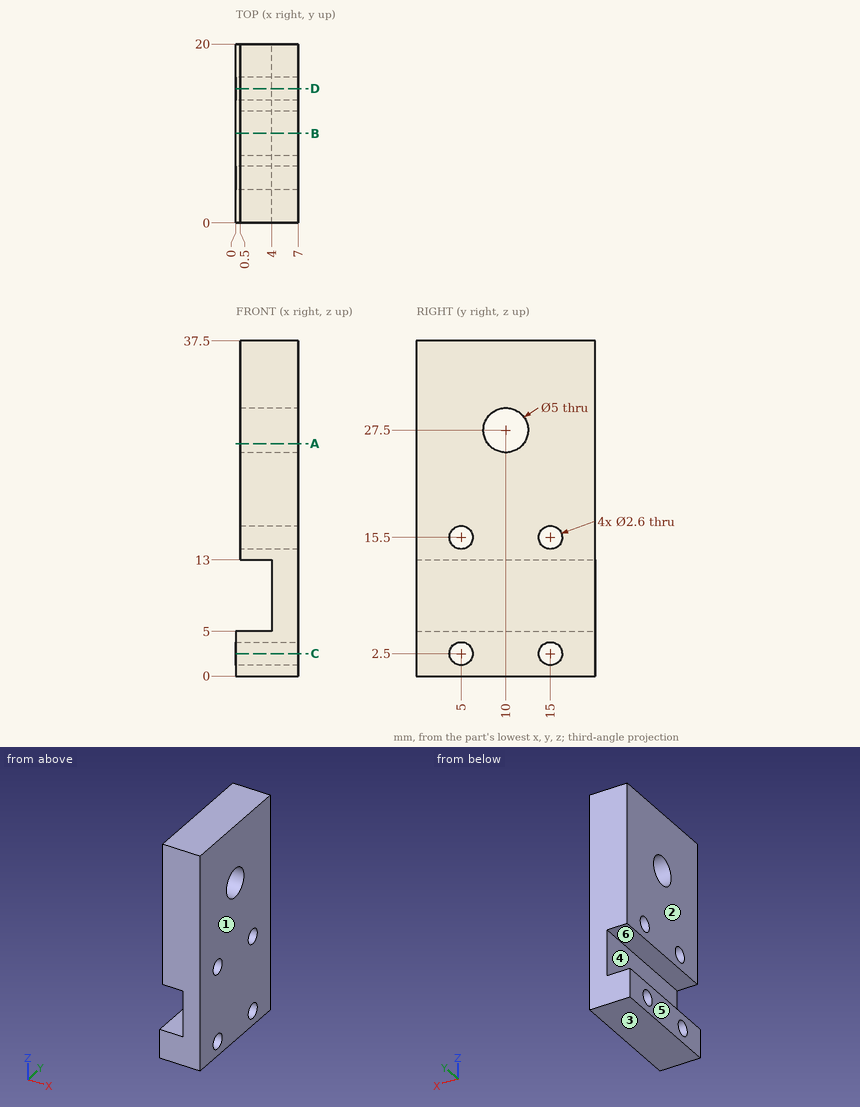
Could you check a few things on this drawing? It's one solid part, dimensions in mm from its lowest x, y, z. A direction names the side the tool comes from. Give positions to 0.01 mm unless a question says otherwise; leave off trailing zeros. Write each loop counter-clockwise with the first axis right and the second up, starting at its lowest first coordinate (ties: lowest second). Pieces come first, ordered by that corner, then holes. Notation, with made-up numbers: M 46,8.25 L 81,8.25 A29 cw 81,41.25 Z; hole C 76,11.5 d1. An arc over 180 degrees is marked long. Put each result on its own line as item: value. Start each with the question number.
Item 1: Thinking about a two-plate mould opening in Z: for the marked faces 3, 4, 5 and 6, which applies, +Z half, -Z half, draft (parallel to the pull), parting line (faces both ways), or undercut?
Item 2: If we section it at B-B, the plane y = 10: Write out the boundary of the cut face in (x, z), then the cut area to 3 significant figures.
Item 3: If we section it at A-A, the plane z = 26: Write out the boundary of the cut face in (x, y), then the cut area to 3 significant figures.
Item 4: On a 3-axis mill with a long thin cutter (end or side, diameter ignored), from which of +Z, -Z, +X, -X, +Y, -Y can I reach the whole of each face in a straight line? I mean the marked faces 1 and 2. Say none if no direction works.
Item 5: If we section it at D-D, the plane y = 15: Write out the boundary of the cut face in (x, z).
Item 6: Will these pins go through, and if not, where does the flat tip stop? pin 1 (8 mm diameter, centred on y = 9, z = 25, fed in from -X); pin 2 (4 mm diameter, centred on y = 12, z = 8, fed in from -X).
Item 7: If we section it at C-C, the plane z = 2.5: Write out the boundary of the cut face in (x, y), then the cut area to 3 significant figures.
Item 8: I need wall thicknesses on L1, parallel to Y at x = 2.5, z = 15.5; L2, parallel to Z at x = 2.25, y = 16.5; L3, parallel to Z at x = 5.25, y = 15.25. Which ranges of each line are inside material? Lowest first, please. Write a range as from..to.
Values:
1. face 3: -Z half
1. face 4: undercut
1. face 5: draft
1. face 6: undercut
2. outline: M 0,0 L 7,0 L 7,25 L 0.5,25 L 0.5,13 L 4,13 L 4,5 L 0,5 Z; M 0.5,30 L 7,30 L 7,37.5 L 0.5,37.5 Z
2. area: 186 mm²
3. outline: M 0.5,0 L 7,0 L 7,8 L 0.5,8 Z; M 0.5,12 L 7,12 L 7,20 L 0.5,20 Z
3. area: 104 mm²
4. face 1: +Z, -Z, +X, +Y, -Y
4. face 2: +Z, -X, +Y, -Y
5. outline: M 0,0 L 7,0 L 7,1.2 L 0,1.2 Z; M 0,3.8 L 7,3.8 L 7,14.2 L 0.5,14.2 L 0.5,13 L 4,13 L 4,5 L 0,5 Z; M 0.5,16.8 L 7,16.8 L 7,37.5 L 0.5,37.5 Z
6. pin 1: x = 0.5
6. pin 2: x = 4
7. outline: M 0,0 L 7,0 L 7,3.7 L 0,3.7 Z; M 0,6.3 L 7,6.3 L 7,13.7 L 0,13.7 Z; M 0,16.3 L 7,16.3 L 7,20 L 0,20 Z
7. area: 104 mm²
8. L1: 0..3.7, 6.3..13.7, 16.3..20
8. L2: 0..5, 13..37.5
8. L3: 0..1.22, 3.78..14.22, 16.78..37.5
